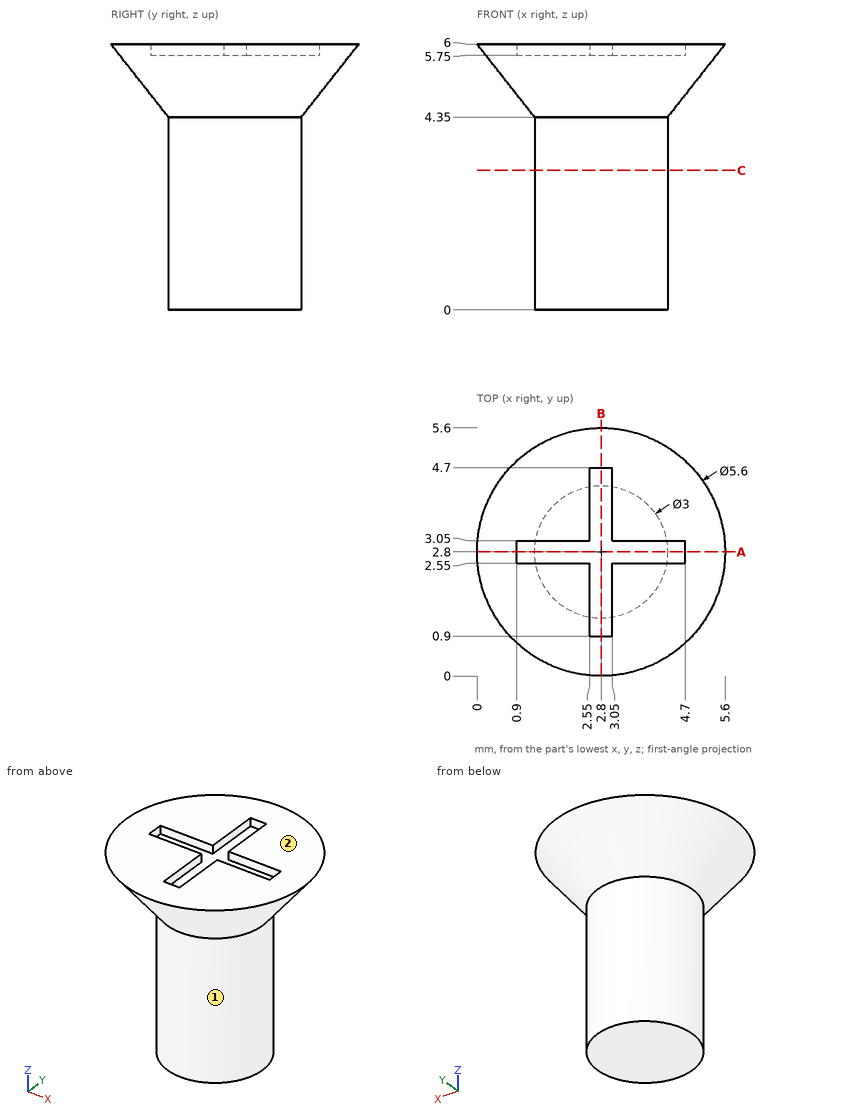
Source: three-view drawing plus pictorial views. Frame: mm from the lowest corner of the part. A direction names the side the tool comes from. Give positions to 0.01 mm unless a question says otherwise; leave off trailing zeros. Order: outer loops, then holes, each group sorted by start corner. A loop starts at its lowest first (then second) coordinate and runs counter-clockwise, first axis right, second up. Notation, with made-up numbers: (33.5, 72.5) -> (60.5, 72.5) arc R13 ccw to (60.5, 87.5) -> close; hole circle Ø8 at (-7.75, 60.25). An arc over 180 degrees is marked (long way). Write each question's results on one line, items separated by ' | '. Start each with the question number.
Item 1: Line query: line 1 (Z direction, x = 2.8, y = 4); line 2 (X direction, y = 2.75, z = 0.85); line 3 (Z direction, x = 1.2, y = 0.9). Output: solid intervals per line, ascending.
Item 2: Cut plane C-C on z = 3.15. Return the cut outline in (x, y).
Item 3: Cut plane A-A on y = 2.8. Return the cut outline in (x, z).
Item 4: Contact query for flat-ended pins moving along their axis: P1, Ø1, axis at x = 5, z = 2.5, coming from the -Y side; P2, Ø1.5, axis at x = 1.5, z = 3.5, coming from the -Y side; P3, Ø1.5, axis at x = 2, z = 2, coming from the +Y side. Output: stop coordinate, or through.
Item 5: Set-up query: the marked faces 1 and 2. Return all of +Z, -Z, +X, -X, +Y, -Y with unobstructed straight access to the full face (end or side cutting, diameter ignored); none if empty.
Established:
1) line 1: 0 to 5.75 | line 2: 1.3 to 4.3 | line 3: 5.6 to 6
2) outline: circle Ø3 at (2.8, 2.8)
3) outline: (0, 6) -> (1.3, 4.35) -> (1.3, 0) -> (4.3, 0) -> (4.3, 4.35) -> (5.6, 6) -> (4.7, 6) -> (4.7, 5.75) -> (0.9, 5.75) -> (0.9, 6) -> close
4) P1: through | P2: y = 1.4 | P3: y = 4.3
5) face 1: -Z | face 2: +Z, +X, -X, +Y, -Y
